Autodesk Inventor part; units mm, degrees
ref_plane "Work Plane1" through (0, 0, 0) normal (0, -1, 0) x (1, 0, 0)
ref_plane "Work Plane2" through (0, 0, -22.86) normal (0, 0, 1) x (1, 0, 0)
ref_plane "YZ Plane" through (0, 0, 0) normal (1, 0, 0) x (0, 1, 0)
sketch "Sketch1" plane through (0, 0, 0) normal (0, 1, 0) x (-1, 0, 0)
  circle A0 centre (0, 0) radius 43.18
  dimension "d0" = 86.36
extrude "Extrusion1" add sketch "Sketch1" against normal blind 63.5
sketch "Sketch2" plane through (0, 0, 0) normal (0, 0, 1) x (1, 0, 0)
  line L0 (-43.18, 0) -> (43.18, 0)
  arc A0 (-43.18, 0) -> (43.18, 0) centre (0, 24.003) ccw
  line L1 (-43.18, -63.5) -> (43.18, -63.5)
  point P0 (0, 0)
  dimension "d4" = 38.1
extrude "Extrusion2" cut sketch "Sketch2" along normal mid plane 101.6
ref_plane "Work Plane1" through (0, 0, 0) normal (0, -1, 0) x (1, 0, 0)
sketch "Sketch3" plane through (0, 0, 0) normal (0, -1, 0) x (1, 0, 0)
  circle A0 centre (0, 0) radius 38.1
  dimension "d8" = 76.2
extrude "Extrusion3" cut sketch "Sketch3" along normal blind 57.15
sketch "Sketch4" plane through (0, 0, 0) normal (1, 0, 0) x (0, 1, 0)
  circle A0 centre (-25.4, 0) radius 12.7
  point P0 (0, 0)
  dimension "d11" = 25.4
  dimension "d12" = 25.4
  dimension "d13" = 0
extrude "Extrusion4" add sketch "Sketch4" along normal mid plane 78.74
sketch "Sketch5" plane through (0, 0, 0) normal (1, 0, 0) x (0, 1, 0)
  circle A0 centre (-25.4, 0) radius 13.97
  arc A1 (-25.4, 17.145) -> (-25.4, -17.145) centre (-25.4, 0) ccw
  line L0 (-63.5, 43.18) -> (-63.5, -43.18)
  circle A2 centre (93.98, 0) radius 20.32
  arc A3 (90.484, -25.1583) -> (93.98, 25.4) centre (93.98, 0) ccw
  line L1 (93.98, 25.4) -> (-25.4, 17.145)
  line L2 (90.484, -25.1583) -> (-25.4, -17.145)
  point P0 (0, 0)
  point P1 (-25.4, 12.7)
  dimension "d16" = 27.94
  dimension "d17" = 34.29
  dimension "d18" = 38.1
  dimension "d19" = 43.18
  dimension "d20" = 40.64
  dimension "d21" = 0
  dimension "d22" = 119.38
  dimension "d23" = 50.8
extrude "Extrusion5" add sketch "Sketch5" along normal mid plane 31.75
sketch "Sketch6" plane through (0, 0, 0) normal (1, 0, 0) x (0, 1, 0)
  circle A0 centre (93.98, 0) radius 20.32 construction
  line L0 (93.98, 0) -> (93.98, -43.5701)
  line L1 (93.98, 0) -> (93.98, 40.9183)
  line L2 (93.98, 40.9183) -> (142.8926, 40.9183)
  line L3 (142.8926, 40.9183) -> (133.2711, -47.8298)
  line L4 (133.2711, -47.8298) -> (93.98, -43.5701)
  point P0 (0, 0)
extrude "Extrusion6" cut sketch "Sketch6" along normal mid plane 2540
ref_plane "Work Plane2" through (0, 0, -22.86) normal (0, 0, 1) x (1, 0, 0)
sketch "Sketch7" plane through (0, 0, -22.86) normal (0, 0, 1) x (1, 0, 0)
  line L0 (15.875, 90.484) -> (15.875, 93.98)
  line L1 (-15.875, -25.4) -> (-15.875, 93.98) construction
  line L2 (15.875, 93.98) -> (-15.875, 93.98)
  line L3 (-15.875, 93.98) -> (-15.875, 88.9)
  line L4 (-15.875, 88.9) -> (15.875, 88.9)
  line L5 (15.875, 88.9) -> (15.875, 93.98)
  point P0 (0, 0)
  dimension "d29" = 5.08
extrude "Extrusion7" add sketch "Sketch7" against normal blind 6.35
mirror "Mirror1" about plane through (0, 0, 0) normal (0, 0, 1) of "Extrusion7"
sketch "Sketch8" plane through (15.875, 0, 0) normal (1, 0, 0) x (0, 0, -1)
  circle A0 centre (0, -25.4) radius 13.97
  line L0 (-20.32, 93.98) -> (-29.21, 93.98)
  arc A1 (-20.32, 93.98) -> (20.32, 93.98) centre (0, 93.98) ccw
  line L1 (20.32, 93.98) -> (29.21, 93.98)
  line L2 (29.21, 88.9) -> (29.21, 93.98)
  line L3 (25.0487, 88.9) -> (29.21, 88.9)
  line L4 (25.0487, 88.9) -> (17.145, -25.4)
  arc A2 (-17.145, -25.4) -> (17.145, -25.4) centre (0, -25.4) ccw
  line L5 (-17.145, -25.4) -> (-25.0487, 88.9)
  line L6 (-25.0487, 88.9) -> (-29.21, 88.9)
  line L7 (-29.21, 88.9) -> (-29.21, 93.98)
  point P0 (0, 0)
extrude "Extrusion8" cut sketch "Sketch8" against normal blind 38.1 keep common part
properties part number "PistonsRod"
Build history of the part. All positions in model axes, mm. A direction names the side the tool comes from. Coordinates: 2 decimals unless noted, no trailing zeros. Write each loop counter-clockwise with the first axis right and the second up, starting at its lowest first coordinate (ties: lowest second). Pieces come first, ordered by that corner, then holes. Notation, with made-up numbers: (-13, 73) -> (20, 73) arc R33 ccw to (20, 106) -> close; hole circle Ø2 at (2.25, 87). An arc over 180 degrees is marked (long way). Use CSV: the item, a comma, the result in double quotes. Start each with the question number.
Q1. Pull direction Z, two halves, no side cores. Call faces 1 (the cylindrical face through (-0.222, 73.665, -0.447)), 2 (the cylindrical face through (-0.22, -42.54, -0.38)), 3 (the flat face through (0, 93.98, -25)), 4 (the flat face through (0.22, 30.95, 21.04)): released by +Z, released by -Z, zero draft, split by the parting line, or undercut.
Q2. Drill centre lines: probe 1 along Z at (x, y) = (-5.5, -25.4) (3 decimals); probe 2 along Z at (x, y) = (-6, -25); probe 3 along Y at (x, z) = (-7, 0) (3 decimals). Where is each one in solid material? Low to high.
Q3. 3-axis set-ups, long thin cutter, end or side, ignore diameter. For faces 5 (the flat face through (0, 88.9, -27)), 6 (the flat face through (0, 91, 29.21)), 7 (the flat face through (0, 88.9, 27)): which of +Z, -Z, +X, -X, +Y, -Y reach the whole face in a straight line?
Q4. Cut at A-A, the plane x = -3. List the corners of the cut face in (y, z) (3 decimals), then the cut area to 3 significant figures.
Q5. Cut at C-C, the plane y = -13.5. List the corners of the cut face in (x, z) (3 decimals).
Q6. Flat gauge pins, fed straight in: pin 1 Ø2 at (x, z) = (-4.5, 28) entering from -Y; pin 2 Ø12 at (x, y) = (-7.5, 2.5) entering from +Z; pin 3 Ø8 at (y, z) = (78.5, 11.5) entering from +X (3 decimals); pin 4 Ø8 at (x, y) = (7, 65.5) entering from +Z. Where does each tip first touch, or does it go through?
Q7. Cut at D-D, the plane y = 16. List the corners of the cut face in (x, z) (3 decimals), then the cut area to 3 significant figures.
Q8. Cut at B-B, the plane z = 0. List the corners of the cut face in (x, y) (3 decimals).
Checked values:
1,face 1,"undercut"
1,face 2,"split by the parting line"
1,face 3,"zero draft"
1,face 4,"released by +Z"
2,probe 1,"z = -17.145 to -13.97, 13.97 to 17.145"
2,probe 2,"z = -17.17 to -13.96, 13.96 to 17.17"
2,probe 3,"y = -42.545 to -39.37, -11.43 to 73.66"
3,face 5,"-Z, +X, -X, -Y"
3,face 6,"+Z, +X, -X, +Y, -Y"
3,face 7,"+Z, +X, -X, -Y"
4,outline,"(-25.4, -17.145) -> (88.9, -25.049) -> (88.9, -29.21) -> (93.98, -29.21) -> (93.98, -20.32) arc R20.32 cw to (93.98, 20.32) -> (93.98, 29.21) -> (88.9, 29.21) -> (88.9, 25.049) -> (-25.4, 17.145) arc R17.145 ccw to start; hole circle Ø27.94 at (-25.4, 0)"
4,area,"4,320 mm²"
5,outline,"(-15.875, -17.968) -> (15.875, -17.968) -> (15.875, -7.318) -> (-15.875, -7.318) -> close; (-15.875, 7.318) -> (15.875, 7.318) -> (15.875, 17.968) -> (-15.875, 17.968) -> close"
6,pin 1,"stops at y = 88.9"
6,pin 2,"stops at z = 19.49"
6,pin 3,"stops at x = 15.875"
6,pin 4,"stops at z = 23.71"
7,outline,"(-15.875, -20.008) -> (15.875, -20.008) -> (15.875, 20.008) -> (-15.875, 20.008) -> close"
7,area,"1,270 mm²"
8,outline,"(-15.875, -42.545) -> (15.875, -42.545) -> (15.875, -39.37) -> (-15.875, -39.37) -> close; (-15.875, -11.43) -> (15.875, -11.43) -> (15.875, 73.66) -> (-15.875, 73.66) -> close"
